CAD build for the part. Positions are in the model's coordinates, mm. A direction names the side the tool comes from. Coordinates: 2 decimals unless noted, no trailing zeros. Order: outer loops, then holes, each group sorted by start corner. A loop starts at its lowest first (then second) coordinate and runs counter-clockwise, first axis right, second up. Notation, with made-up numbers: (-9, 66) - (36, 66) arc R22 cw to (36, 104) - close; hole circle Ø1 at (66.25, 83). An arc over 180 degrees is marked (long way). Return JSON: item names as keys, results as strings.
from build123d import *
from OCP.BRepFilletAPI import BRepFilletAPI_MakeChamfer

# Parameters (mm, degrees)
SKETCH1_W           = 16
SKETCH1_H           = 16
BOSS_EXTRUDE1_DEPTH = 10
CUT_EXTRUDE1_DEPTH  = 1
FILLET4_SIZE        = 2
FILLET4_SIZE2       = 1.2


with BuildPart() as part:
    # Sketch1 → Boss-Extrude1 (new body)
    with BuildSketch(Plane.XY):
        with Locations((8, 8)):
            Rectangle(SKETCH1_W, SKETCH1_H)
    extrude(amount=BOSS_EXTRUDE1_DEPTH)

    # Sketch2 → Cut-Extrude1 (cut)
    with BuildSketch(Plane.XY.offset(10)):
        Polygon((4.316390203, 12.684359808), (4.285030305, 3.333745838), (12.398579492, 7.981894354), align=None)
    extrude(amount=-CUT_EXTRUDE1_DEPTH, mode=Mode.SUBTRACT)

    # Fillet4: one chamfer whose edges measure the first distance from different faces: ONE call of the kernel's chamfer builder (chamfer() names one face for all edges)
    fillet4_edges_1 = [part.edges().sort_by_distance(p)[0] for p in [
        (16, 8, 10),
    ]]
    fillet4_side_1 = [part.faces().sort_by_distance(p)[0] for p in [
        (16, 8, 5),
    ]]
    fillet4_edges_2 = [part.edges().sort_by_distance(p)[0] for p in [
        (8, 16, 10),
    ]]
    fillet4_side_2 = [part.faces().sort_by_distance(p)[0] for p in [
        (8, 16, 5),
    ]]
    fillet4_edges_3 = [part.edges().sort_by_distance(p)[0] for p in [
        (0, 8, 10),
    ]]
    fillet4_side_3 = [part.faces().sort_by_distance(p)[0] for p in [
        (0, 8, 5),
    ]]
    fillet4_edges_4 = [part.edges().sort_by_distance(p)[0] for p in [
        (8, 0, 10),
    ]]
    fillet4_side_4 = [part.faces().sort_by_distance(p)[0] for p in [
        (8, 0, 5),
    ]]
    fillet4 = BRepFilletAPI_MakeChamfer(part.part.solid().wrapped)
    for e in fillet4_edges_1:
        fillet4.Add(FILLET4_SIZE, FILLET4_SIZE2, e.wrapped, fillet4_side_1[0].wrapped)  # the first distance lies on this face
    for e in fillet4_edges_2:
        fillet4.Add(FILLET4_SIZE, FILLET4_SIZE2, e.wrapped, fillet4_side_2[0].wrapped)  # the first distance lies on this face
    for e in fillet4_edges_3:
        fillet4.Add(FILLET4_SIZE, FILLET4_SIZE2, e.wrapped, fillet4_side_3[0].wrapped)  # the first distance lies on this face
    for e in fillet4_edges_4:
        fillet4.Add(FILLET4_SIZE, FILLET4_SIZE2, e.wrapped, fillet4_side_4[0].wrapped)  # the first distance lies on this face
    add(Compound.cast(fillet4.Shape()), mode=Mode.REPLACE)


solid = part.part
Item 1: Band-saw the part on C-C, the plane z = 8.5. List the corners of the cut face in (x, y).
Findings below:
{"outline": "(0.3, 0.3) - (15.7, 0.3) - (15.7, 15.7) - (0.3, 15.7) - close"}
Item 2: Band-saw the part on B-B, the plane x = 10.25. List the corners of the cut face in (y, z).
Findings below:
{"outline": "(0, 0) - (16, 0) - (16, 8) - (14.8, 10) - (9.23, 10) - (9.23, 9) - (6.75, 9) - (6.75, 10) - (1.2, 10) - (0, 8) - close"}
Item 3: Drop flat-ended pins along their axis: P1, Ø3, axis at x = 9, z = 3.5, coming from the -Y side; P2, Ø1.5, axis at x = 11.5, z = 9, coming from the +Y side. Give the stop position or say it passes through.
Findings below:
{"P1": "stops at y = 0", "P2": "stops at y = 15.85"}
Item 4: Wall check: L1, parallel to X at y = 12, z = 9.75; L2, parallel to Z at x = 4.5, y = 9.5; L3, parallel to Y at x = 3, z = 8.75. Give the ranges that are in metal, low to high. Write a range as [from, to].
Findings below:
{"L1": "x = [1.05, 4.31], [5.49, 14.95]", "L2": "z = [0, 9]", "L3": "y = [0.45, 15.55]"}
Item 5: Which spindle directions (+Z, -Z, +X, -X, +Y, -Y) get a long thin tool onto all of the face, cutting with end or side? Do faces 1 (the flat face through (8.414, 10.3, 9.507)), 2 (the flat face through (0, 8, 4)). Say none if no direction does.
Findings below:
{"face 1": "+Z", "face 2": "+Z, -Z, -X, +Y, -Y"}
Item 6: Mould opens along Y. For faces 3 (the flat face through (8.29, 5.63, 9.51)), 4 (the flat face through (8, 0, 4)), 5 (the flat face through (16, 8, 4)) say: released by +Y, released by -Y, zero draft, split by the parting line, or undercut.
Findings below:
{"face 3": "undercut", "face 4": "released by -Y", "face 5": "zero draft"}
Item 7: Band-saw the part on D-D, the plane x = 1.5. List the corners of the cut face in (y, z).
Findings below:
{"outline": "(0, 0) - (16, 0) - (16, 8) - (14.8, 10) - (1.2, 10) - (0, 8) - close"}
Item 8: Band-saw the part on A-A, the plane y = 8.5. List the corners of the cut face in (x, z), then the cut area to 3 significant figures.
Findings below:
{"outline": "(0, 0) - (16, 0) - (16, 8) - (14.8, 10) - (11.51, 10) - (11.51, 9) - (4.3, 9) - (4.3, 10) - (1.2, 10) - (0, 8) - close", "area": "150 mm²"}
